from build123d import *

# Parameters (mm, degrees)
BODY_DEPTH             = 3
MAGNET_CUTOUT_SKETCH_W = 2.2
MAGNET_CUTOUT_SKETCH_H = 6.2
MAGNET_CUTOUT_DEPTH    = 2.6
BORDER_DEPTH           = 0.5
FILLET_1_R             = 1.5


with BuildPart() as part:
    # surface_sketch → body (new body)
    with BuildSketch(Plane(origin=(0, 0, 0), x_dir=(1, 0, 0), z_dir=(0, 1, 0))):
        Polygon((-12.4, -15), (10.1, -15), (10.1, 15), (-8.4, 15), (-12.4, 11), align=None)
    extrude(amount=-BODY_DEPTH)

    # magnet_cutout_sketch → magnet_cutout (cut)
    with BuildSketch(Plane.XZ.offset(3)):
        with Locations((9, 0)):
            Rectangle(MAGNET_CUTOUT_SKETCH_W, MAGNET_CUTOUT_SKETCH_H)
    magnet_cutout = extrude(amount=-MAGNET_CUTOUT_DEPTH, mode=Mode.SUBTRACT)

    # magnet_cutout_mirror: magnet_cutout across plane
    add(magnet_cutout.mirror(Plane(origin=(-1.15, 0, 0), x_dir=(0, 0, 1), z_dir=(1, 0, 0))), mode=Mode.SUBTRACT)

    # border_sketch → border (add)
    with BuildSketch(Plane(origin=(0, 0, 0), x_dir=(1, 0, 0), z_dir=(0, 1, 0))):
        with BuildLine():
            Line((-7.778679656, 15), (8.6, 15))
            ThreePointArc((8.6, 15), (9.660660172, 14.560660172), (10.1, 13.5))
            Line((10.1, 13.5), (10.1, -13.571428571))
            ThreePointArc((10.1, -13.571428571), (9.660660172, -14.632088743), (8.6, -15.071428571))
            Line((8.6, -15.071428571), (-10.9, -15.071428571))
            ThreePointArc((-10.9, -15.071428571), (-11.960660172, -14.632088743), (-12.4, -13.571428571))
            Line((-12.4, -13.571428571), (-12.4, 10.378679656))
            ThreePointArc((-12.4, 10.378679656), (-12.285819299, 10.952704805), (-11.960660172, 11.439339828))
            Line((-11.960660172, 11.439339828), (-8.839339828, 14.560660172))
            ThreePointArc((-8.839339828, 14.560660172), (-8.352704805, 14.885819299), (-7.778679656, 15))
        make_face()
        with BuildLine():
            Line((-7.778679656, 14), (8.6, 14))
            ThreePointArc((8.6, 14), (8.953553391, 13.853553391), (9.1, 13.5))
            Line((9.1, 13.5), (9.1, -13.571428571))
            ThreePointArc((9.1, -13.571428571), (8.953553391, -13.924981962), (8.6, -14.071428571))
            Line((8.6, -14.071428571), (-10.9, -14.071428571))
            ThreePointArc((-10.9, -14.071428571), (-11.253553391, -13.924981962), (-11.4, -13.571428571))
            Line((-11.4, -13.571428571), (-11.4, 10.378679656))
            ThreePointArc((-11.4, 10.378679656), (-11.361939766, 10.570021373), (-11.253553391, 10.732233047))
            Line((-11.253553391, 10.732233047), (-8.132233047, 13.853553391))
            ThreePointArc((-8.132233047, 13.853553391), (-7.970021373, 13.961939766), (-7.778679656, 14))
        make_face(mode=Mode.SUBTRACT)
    extrude(amount=BORDER_DEPTH)

    # Скругление1
    # the kernel refuses this fillet: 1.5 mm, written as the material it takes off along each edge
    with BuildSketch(Plane(origin=(10.1, 3.75, 15), x_dir=(-1, 0, 0), z_dir=(0, -1, 0))) as fillet_1_piece_1_section:
        with BuildLine():
            CenterArc((FILLET_1_R, FILLET_1_R), FILLET_1_R, 180, 90)
            Line((0, FILLET_1_R), (0, 0))
            Line((0, 0), (FILLET_1_R, 0))
        make_face()
    fillet_1_piece_1 = extrude(amount=10.5, mode=Mode.PRIVATE)
    fillet_1_piece_1 = fillet_1_piece_1 - Plane(origin=(8.6, 0.25, 13.571428571), x_dir=(1, 0, 0), z_dir=(0, -1, 0)) * Cylinder(1.5, 27, mode=Mode.PRIVATE)
    add(fillet_1_piece_1, mode=Mode.SUBTRACT)
    with BuildSketch(Plane(origin=(10.1, 0, 15), x_dir=(-1, 0, 0), z_dir=(0, -1, 0))) as fillet_1_piece_2:
        with BuildLine():
            CenterArc((FILLET_1_R, FILLET_1_R), FILLET_1_R, 180, 90)
            Line((0, FILLET_1_R), (0, 0))
            Line((0, 0), (FILLET_1_R, 0))
        make_face()
    extrude(amount=6.75, mode=Mode.SUBTRACT)
    with BuildSketch(Plane(origin=(10.1, 3.75, -15), x_dir=(0, 0, 1), z_dir=(0, -1, 0))) as fillet_1_piece_3:
        with BuildLine():
            CenterArc((FILLET_1_R, FILLET_1_R), FILLET_1_R, 180, 90)
            Line((0, FILLET_1_R), (0, 0))
            Line((0, 0), (FILLET_1_R, 0))
        make_face()
    extrude(amount=10.5, mode=Mode.SUBTRACT)
    with BuildSketch(Plane(origin=(-12.4, 3.75, 15), x_dir=(1, 0, 0), z_dir=(0, -1, 0))) as fillet_1_piece_4_section:
        with BuildLine():
            CenterArc((FILLET_1_R, -FILLET_1_R), FILLET_1_R, 90, 90)
            Line((0, -FILLET_1_R), (0, 0))
            Line((0, 0), (FILLET_1_R, 0))
        make_face()
    fillet_1_piece_4 = extrude(amount=10.5, mode=Mode.PRIVATE)
    fillet_1_piece_4 = fillet_1_piece_4 - Plane(origin=(-10.9, 0.25, 13.571428571), x_dir=(0, 0, 1), z_dir=(0, -1, 0)) * Cylinder(1.5, 27, mode=Mode.PRIVATE)
    add(fillet_1_piece_4, mode=Mode.SUBTRACT)
    with BuildSketch(Plane(origin=(-12.4, 0, 15), x_dir=(1, 0, 0), z_dir=(0, -1, 0))) as fillet_1_piece_5:
        with BuildLine():
            CenterArc((FILLET_1_R, -FILLET_1_R), FILLET_1_R, 90, 90)
            Line((0, -FILLET_1_R), (0, 0))
            Line((0, 0), (FILLET_1_R, 0))
        make_face()
    extrude(amount=6.75, mode=Mode.SUBTRACT)
    with BuildSketch(Plane(origin=(-8.4, 1.553300859, -15), x_dir=(-0.7071067811865476, 0, 0.7071067811865476), z_dir=(0, -1, 0)), Plane(origin=(-12.4, 1.553300859, -11), x_dir=(0, 0, 1), z_dir=(0, -1, 0))) as fillet_1_piece_6:
        with BuildLine():
            CenterArc((FILLET_1_R * 0.414213562373, -FILLET_1_R), FILLET_1_R, 90, 45)
            Line((-FILLET_1_R * 0.292893218813, -FILLET_1_R * 0.292893218813), (0, 0))
            Line((0, 0), (FILLET_1_R * 0.414213562373, 0))
        make_face()
    extrude(amount=6.106601718, mode=Mode.SUBTRACT)


solid = part.part
Could you check a few things on this model? Use its own coordinates, in mm. A direction names the side the tool comes from. Give positions to 0.01 mm unless a question says otherwise; leave off trailing zeros. Order: outer loops, then holes, each group sorted by start corner. A loop starts at its lowest first (then second) coordinate and runs counter-clockwise, first axis right, second up.
1. I need wall thicknesses on L1, parallel to X at y = 0.1, z = 2.5; L2, parallel to Z at x = -2.75, y = 0.35; L3, parallel to X at y = -1.6, z = -2. Which ranges of each line are inside material? Lowest first, please.
2. Suppose I cut it at B-B (z = -3.5). List the corners of the cut face in (x, y) for me.
3. Suppose I cut it at A-A (x = 4.5). List the corners of the cut face in (y, z) for me.
4. We'd pull the mould along Z, two halves only. Please class faces 5 (the cylindrical face through (-11.95, -1.61, 14.57)), 6 (the cylindrical face through (-8.36, -1.226, -14.883)), 7 (the flat face through (-10.2, -2, 0)): pulls with the +Z half, pulls with the -Z half, needs draft (parallel to the pull), parting line crosses it, or undercut.
5. Will these pins go through, and if not, where does the flat tip stop? P1, Ø10, axis at x = -3, z = 4, coming from the +Y side; P2, Ø1.1, axis at x = -11, y = -1.5, coming from the -Z side; P3, Ø1.1, axis at x = -11, y = -2.5, coming from the +Z side.
6. For faces 1 (the flat face through (-1, -1, 15)), 2 (the flat face through (-1, 0, 0)), 3 (the flat face through (-11, -2, -3.1)), 4 (the flat face through (9, -2, -3.1)), which set-ups out of +Z, -Z, +X, -X, +Y, -Y let a thin tool reach every point of the face, with its end or its side?
7. Suppose I cut it at C-C (y = -2.2). List the corners of the cut face in (x, z) for me, plus the area to 3 significant figures.
Solved:
1. L1: x = -12.4 to -11.4, 9.1 to 10.1
1. L2: z = -15 to -14, 14.07 to 15.07
1. L3: x = -10.2 to 7.9
2. outline: (-12.4, -3) - (10.1, -3) - (10.1, 0.5) - (9.1, 0.5) - (9.1, 0) - (-11.4, 0) - (-11.4, 0.5) - (-12.4, 0.5) - close
3. outline: (-3, -15) - (0.5, -15) - (0.5, -14) - (0, -14) - (0, 14.07) - (0.5, 14.07) - (0.5, 15.07) - (0, 15.07) - (0, 15) - (-3, 15) - close
4. face 5: pulls with the +Z half
4. face 6: pulls with the -Z half
4. face 7: undercut
5. P1: stops at y = 0
5. P2: stops at z = -12.95
5. P3: stops at z = 15
6. face 1: +Z, +X, -X, -Y
6. face 2: +Y
6. face 3: -X, -Y
6. face 4: +X, -Y
7. outline: (-12.4, -10.38) arc R1.5 ccw to (-11.96, -11.44) - (-8.84, -14.56) arc R1.5 ccw to (-7.78, -15) - (8.6, -15) arc R1.5 ccw to (10.1, -13.5) - (10.1, -3.1) - (7.9, -3.1) - (7.9, 3.1) - (10.1, 3.1) - (10.1, 13.5) arc R1.5 ccw to (8.6, 15) - (-10.9, 15) arc R1.5 ccw to (-12.4, 13.5) - (-12.4, 3.1) - (-10.2, 3.1) - (-10.2, -3.1) - (-12.4, -3.1) - close
7. area: 638 mm2
